Geometry: see drawing. Coordinates: mm, zero at the bounding-box minimum. Coordinates: 2 decimals unless noted, no trailing zeros. Write each loop counter-clockwise with the first axis right and the second up, starting at its lowest first coordinate (ties: lowest second). Pieces come first, ordered by that corner, then holes.
1) Section query B-B (z = 3.5). Output: boundary loops of the cut face in (x, y), then the cut area to 3 significant figures.
2) Draft query along X for the marked faces 1, 2 and 3. Return one class per face: pulls with the +X half, pulls with the -X half, needs draft (parallel to the pull), parting line crosses it, or undercut.
3) Line query: L1, parallel to Y at x = 12, z = 5.75; L2, parallel to X at y = 11.75, z = 2.75; L3, parallel to Y at x = 14.5, z = 9.5. Output: solid intervals per line, ascending.
4) Pin query (flat end, axial travel): pin 1 Ø5 at (x, z) = (19.5, 4.5) entering from -Y; pin 2 Ø1.5 at (y, z) = (7, 5) entering from -X; pin 3 Ø6 at (y, z) = (3, 3) entering from -X. Return the tip coordinate at first contact, or that it passes through.
5) Section query A-A (y = 12). Output: boundary loops of the cut face in (x, z).
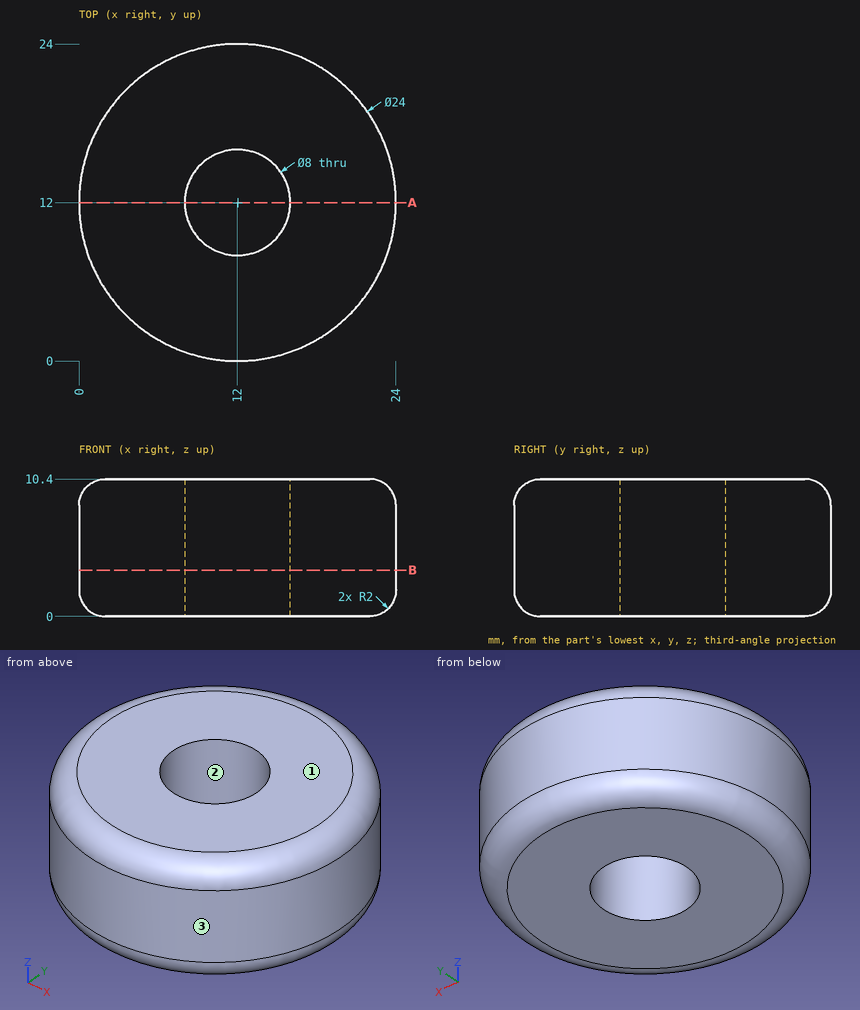
Answer:
1. outline: circle Ø24 at (12, 12); hole circle Ø8 at (12, 12)
1. area: 402 mm2
2. face 1: needs draft
2. face 2: undercut
2. face 3: parting line crosses it
3. L1: y = 0 to 8, 16 to 24
3. L2: x = 0 to 8.01, 15.99 to 24
3. L3: y = 0.6 to 8.88, 15.12 to 23.4
4. pin 1: stops at y = 1.09
4. pin 2: stops at x = 0.78
4. pin 3: stops at x = 1.61
5. outline: (0, 2) arc R2 ccw to (2, 0) - (8, 0) - (8, 10.4) - (2, 10.4) arc R2 ccw to (0, 8.4) - close; (16, 0) - (22, 0) arc R2 ccw to (24, 2) - (24, 8.4) arc R2 ccw to (22, 10.4) - (16, 10.4) - close
